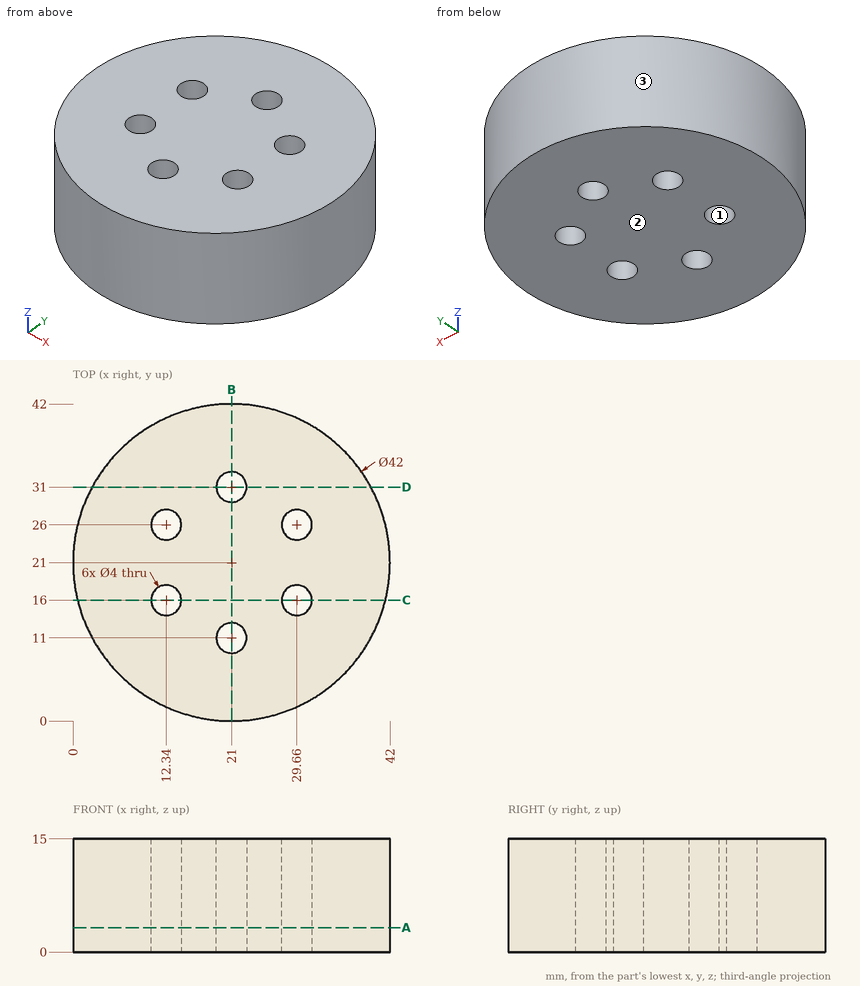
Check sheet for the drawn part. Datum: minimum x, y, z corner. Units: mm. Round coordinates to 2 decimals unless told otherwise and drop trailing zeros. Order: outer loops, then holes, each group sorted by start corner. A loop starts at its lowest first (then second) coordinate and runs counter-clockwise, first axis right, second up.
(1) Scan lines: probe 1 along Y at (x, z) = (20, 6.75); probe 2 along Y at (x, z) = (28.5, 7) (1 decimal); probe 3 along X at (y, z) = (35, 13). Record each from-to range of solid material in increasing order.
(2) Go/stop test with flat-tipped pins: P1, Ø3, axis at y = 13.5, z = 13, coming from the +X side (1 decimal); P2, Ø1.5, axis at y = 12, z = 7.5, coming from the +X side; P3, Ø4, axis at x = 30, z = 5.5, coming from the +Y side. Record where each tip stops, or that it passes through.
(3) Cross-section at B-B, the plane x = 21. Enter the section's corners in (y, z).
(4) Cross-section at C-C, the plane y = 16. Enter the section's corners in (x, z), and give its area (3 significant figures).
(5) Cross-section at D-D, the plane y = 31. Enter the section's corners in (x, z).
(6) Draft check along X on the marked faces 1, 2 and 3. Enter one of: pulls with the +X half, pulls with the -X half, needs draft (parallel to the pull), parting line crosses it, or undercut.
(7) Cross-section at A-A, the plane z = 3.25. Enter the section's corners in (x, y), and give its area (3 significant figures).
Check sheet entries:
1. probe 1: y = 0.02 to 9.27, 12.73 to 29.27, 32.73 to 41.98
1. probe 2: y = 1.4 to 14.4, 17.6 to 24.4, 27.6 to 40.6
1. probe 3: x = 5.35 to 36.65
2. P1: stops at x = 41.1
2. P2: stops at x = 40.31
2. P3: stops at y = 40.8
3. outline: (0, 0) - (9, 0) - (9, 15) - (0, 15) - close; (13, 0) - (29, 0) - (29, 15) - (13, 15) - close; (33, 0) - (42, 0) - (42, 15) - (33, 15) - close
4. outline: (0.6, 0) - (10.34, 0) - (10.34, 15) - (0.6, 15) - close; (14.34, 0) - (27.66, 0) - (27.66, 15) - (14.34, 15) - close; (31.66, 0) - (41.4, 0) - (41.4, 15) - (31.66, 15) - close
4. area: 492 mm2
5. outline: (2.53, 0) - (19, 0) - (19, 15) - (2.53, 15) - close; (23, 0) - (39.47, 0) - (39.47, 15) - (23, 15) - close
6. face 1: undercut
6. face 2: needs draft
6. face 3: parting line crosses it
7. outline: circle Ø42 at (21, 21); hole circle Ø4 at (12.34, 16); hole circle Ø4 at (12.34, 26); hole circle Ø4 at (21, 11); hole circle Ø4 at (21, 31); hole circle Ø4 at (29.66, 16); hole circle Ø4 at (29.66, 26)
7. area: 1,310 mm2
